```python
from build123d import *

# Parameters (mm, degrees)
F0_W     = 4
F0_H     = 10
F0_W_2   = 5
F0_H_2   = 12
F1_DEPTH = 40
F3_R     = 1.99999
F4_D     = 5.2
F4_DEPTH = 12
F4_TIP   = 1.5622376095
F6_D     = 4.2
F6_DEPTH = 12
F6_TIP   = 1.2618073


# Not quite as in the source:
# - a fillet or chamfer is up to 0.001 mm smaller than in the source, because OpenCascade refuses the exact size


with BuildPart() as f1:
    # F0 (on Top) → F1 (new body)
    with BuildSketch(Plane.XY):
        Polygon((-36.5682695345, 36.2048765272), (-76.5682695345, 36.2048765272), (-76.5682695345, 32.2048765272), (-72.5682695345, 32.2048765272), (-41.5682695345, 32.2048765272), (-36.5682695345, 32.2048765272), align=None)
        with Locations((-74.5682695345, 27.2048765272)):
            Rectangle(F0_W, F0_H)
        with Locations((-39.0682695345, 26.2048765272)):
            Rectangle(F0_W_2, F0_H_2)
    extrude(amount=F1_DEPTH)

    # F3 (radius 2 in the source; OpenCascade refuses exactly that, so slightly less here)
    f3_edges = [f1.edges().sort_by_distance(p)[0] for p in [
        (-76.56827, 36.204877, 20),
        (-72.56827, 32.204877, 20),
        (-76.56827, 22.204877, 20),
        (-72.56827, 22.204877, 20),
    ]]
    fillet(f3_edges, radius=F3_R)

    # F4
    with Locations(Plane.YZ.offset(-36.5682695345)):
        with Locations((28.2048765272, 10), (28.2048765272, 30)):
            Hole(F4_D / 2, depth=F4_DEPTH)
            with Locations((0, 0, -(F4_DEPTH + F4_TIP / 2))):  # 118° drill point
                Cone(0, F4_D / 2, F4_TIP, mode=Mode.SUBTRACT)

    # F6
    with Locations(Plane(origin=(0, 36.2048765272, 0), x_dir=(-1, 0, 0), z_dir=(0, 1, 0))):
        with Locations((64.5682695345, 10), (64.5682695345, 30)):
            Hole(F6_D / 2, depth=F6_DEPTH)
            with Locations((0, 0, -(F6_DEPTH + F6_TIP / 2))):  # 118° drill point
                Cone(0, F6_D / 2, F6_TIP, mode=Mode.SUBTRACT)


solid = f1.part
```
Model file for the job. Use its own axes, mm. A direction names the side the tool comes from. Round coordinates to 2 decimals unless told otherwise and drop trailing zeros. Order: outer loops, then holes, each group sorted by start corner. A loop starts at its lowest first (then second) coordinate and runs counter-clockwise, first axis right, second up. Notation, with made-up numbers: (-32, 41) -> (-28, 41) arc R26 ccw to (-28, 79) -> close; hole circle Ø3 at (36.25, 36.25). An arc over 180 degrees is marked (long way). Use one line per item in the form item = value.
Item 1: Cut at B-B, the plane y = 27.5. Write the cut outline in (x, z), and give its area (3 significant figures).
Returned:
outline = (-76.57, 0) -> (-72.57, 0) -> (-72.57, 40) -> (-76.57, 40) -> close; (-41.57, 0) -> (-36.57, 0) -> (-36.57, 7.5) -> (-41.57, 7.5) -> close; (-41.57, 12.5) -> (-36.57, 12.5) -> (-36.57, 27.5) -> (-41.57, 27.5) -> close; (-41.57, 32.5) -> (-36.57, 32.5) -> (-36.57, 40) -> (-41.57, 40) -> close
area = 310 mm^2
Item 2: Pull direction X, two halves, no side cores. Call faces 1 (the face through (-39.1, 30.27, 8.42)), 2 (the face through (-36.568, 28, 20)), 3 (the face through (-72.568, 27, 20)), 4 (the face through (-66.666, 34.177, 30.092)): released by +X, released by -X, zero draft, split by the parting line, or undercut.
Returned:
face_1 = zero draft
face_2 = released by +X
face_3 = undercut
face_4 = undercut
Item 3: Flat gauge pins, fed straight in: pin 1 Ø5 at (x, y) = (-69.5, 24) entering from +Z; pin 2 Ø14.5 at (x, z) = (-49.5, 29.5) entering from -Y. Where does each tip first touch, or does it go through?
Returned:
pin_1 = through
pin_2 = 32.2
Item 4: Tool access for faces 5 (the face through (-39.103, 30.802, 30.114)), 6 (the face through (-56, 32.205, 20)), 7 (the face through (-66.666, 34.177, 10.092)): list every direction of +Z, -Z, +X, -X, +Y, -Y with a clear straight run to the whole face (end or side of a thin tool).
Returned:
face_5 = +X
face_6 = +Z, -Z, -Y
face_7 = +Y, -Y
Item 5: Cut at C-C, the plane y = 31.5. Write the cut outline in (x, z), and give its area (3 significant figures).
Returned:
outline = (-76.57, 0) -> (-72.09, 0) -> (-72.09, 40) -> (-76.57, 40) -> close; (-41.57, 0) -> (-36.57, 0) -> (-36.57, 40) -> (-41.57, 40) -> close
area = 379 mm^2
Item 6: Drill centre lines: line 1 (X direction, y = 28, z = 2); line 2 (Y direction, x = -60, z = 11); line 3 (X direction, y = 21.5, z = 14). Where is each one in solid material? Low to high.
Returned:
line_1 = -76.57 to -72.57, -41.57 to -36.57
line_2 = 32.2 to 36.2
line_3 = -41.57 to -36.57
Item 7: Cut at A-A, the plane z = 10. Give the number of separate pieces and of enclosed holes in the cut face, and give its area (3 significant figures).
Returned:
separate_pieces = 3
enclosed_holes = 0
area = 215 mm^2
